```python
from build123d import *

# Parameters (mm, degrees)
SKETCH1_W               = 666.75
SKETCH1_H               = 117.602
BOSS_EXTRUDE1_DEPTH     = 1.5875
CUT_EXTRUDE1_REACH      = 679.044
SKETCH3_W               = 3.175
SKETCH3_H               = 50.8
CUT_EXTRUDE2_DEPTH      = 678.043804388
FILLET1_R               = 2.54
FILLET1_OF_MIRROR1_R    = 2.54
CUT_EXTRUDE3_DEPTH      = 678.043804388
CUT_EXTRUDE3_DEPTH_BACK = 678.043804388
FILLET2_R               = 2.54
CUT_EXTRUDE4_REACH      = 679.044
BOSS_EXTRUDE7_DEPTH     = 1.5875
CUT_EXTRUDE5_REACH      = 679.044
FILLET3_R               = 2.54
BOSS_EXTRUDE9_DEPTH     = 1.5875
CUT_EXTRUDE10_REACH     = 679.044
FILLET4_R               = 2.54
FILLET5_R               = 17.78


with BuildPart() as part:
    # Sketch1 → Boss-Extrude1 (new body)
    with BuildSketch(Plane.XY):
        with Locations((333.375, 58.801)):
            Rectangle(SKETCH1_W, SKETCH1_H)
    extrude(amount=BOSS_EXTRUDE1_DEPTH)

    # Sketch3 → Cut-Extrude1 (cut, up to next)
    with BuildSketch(Plane(origin=(0, 0, 0), x_dir=(-1, 0, 0), z_dir=(0, 0, -1)), mode=Mode.PRIVATE) as cut_extrude1_sk1:
        with Locations((-215.646, 58.801)):
            Rectangle(SKETCH3_W, SKETCH3_H)
    cut_extrude1_tool1 = extrude(cut_extrude1_sk1.sketch, amount=-CUT_EXTRUDE1_REACH, mode=Mode.PRIVATE) & part.part
    # Sketch3 → Cut-Extrude1 (cut, up to next)
    with BuildSketch(Plane(origin=(0, 0, 0), x_dir=(-1, 0, 0), z_dir=(0, 0, -1)), mode=Mode.PRIVATE) as cut_extrude1_sk2:
        with Locations((-451.104, 58.801)):
            Rectangle(SKETCH3_W, SKETCH3_H)
    cut_extrude1_tool2 = extrude(cut_extrude1_sk2.sketch, amount=-CUT_EXTRUDE1_REACH, mode=Mode.PRIVATE) & part.part
    # Sketch3 → Cut-Extrude1 (cut, up to next)
    with BuildSketch(Plane(origin=(0, 0, 0), x_dir=(-1, 0, 0), z_dir=(0, 0, -1)), mode=Mode.PRIVATE) as cut_extrude1_sk3:
        with Locations((-665.1625, 58.801)):
            Rectangle(SKETCH3_W, SKETCH3_H)
    cut_extrude1_tool3 = extrude(cut_extrude1_sk3.sketch, amount=-CUT_EXTRUDE1_REACH, mode=Mode.PRIVATE) & part.part
    # Sketch3 → Cut-Extrude1 (cut, up to next)
    with BuildSketch(Plane(origin=(0, 0, 0), x_dir=(-1, 0, 0), z_dir=(0, 0, -1)), mode=Mode.PRIVATE) as cut_extrude1_sk4:
        with Locations((-1.5875, 58.801)):
            Rectangle(SKETCH3_W, SKETCH3_H)
    cut_extrude1_tool4 = extrude(cut_extrude1_sk4.sketch, amount=-CUT_EXTRUDE1_REACH, mode=Mode.PRIVATE) & part.part
    add(cut_extrude1_tool1.solids().sort_by_distance((215.646, 58.801, 0))[0], mode=Mode.SUBTRACT)
    add(cut_extrude1_tool2.solids().sort_by_distance((451.104, 58.801, 0))[0], mode=Mode.SUBTRACT)
    add(cut_extrude1_tool3.solids().sort_by_distance((665.1625, 58.801, 0))[0], mode=Mode.SUBTRACT)
    add(cut_extrude1_tool4.solids().sort_by_distance((1.5875, 58.801, 0))[0], mode=Mode.SUBTRACT)

    # Sketch4 → Cut-Extrude2 (cut, symmetric)
    with BuildSketch(Plane(origin=(0, 0, 0), x_dir=(-1, 0, 0), z_dir=(0, 0, -1))):
        Polygon((-482.510180694, 104.902), (-633.756319306, 104.902), (-558.13325, 67.310525631), align=None)
        Polygon((-465.3915, 96.392474369), (-465.3915, 21.209525631), (-541.014569306, 58.801), align=None)
        Polygon((-482.510180694, 12.7), (-633.756319306, 12.7), (-558.13325, 50.291474369), align=None)
        Polygon((-650.875, 96.392474369), (-650.875, 21.209525631), (-575.251930694, 58.801), align=None)
    cut_extrude2 = extrude(amount=CUT_EXTRUDE2_DEPTH, both=True, mode=Mode.SUBTRACT)

    # Fillet1
    fillet1_edges = [part.edges().sort_by_distance(p)[0] for p in [
        (650.875, 21.209525631, 0.79375),
        (650.875, 96.392474369, 0.79375),
        (633.756319306, 12.7, 0.79375),
        (558.13325, 50.291474369, 0.79375),
        (482.510180694, 12.7, 0.79375),
        (482.510180694, 104.902, 0.79375),
        (558.13325, 67.310525631, 0.79375),
        (633.756319306, 104.902, 0.79375),
        (541.014569306, 58.801, 0.79375),
        (465.3915, 96.392474369, 0.79375),
        (465.3915, 21.209525631, 0.79375),
        (575.251930694, 58.801, 0.79375),
    ]]
    fillet(fillet1_edges, radius=FILLET1_R)

    # Mirror1: Cut-Extrude2 across plane
    add(cut_extrude2.mirror(Plane(origin=(333.375, 0, 0), x_dir=(0, 0, 1), z_dir=(1, 0, 0))), mode=Mode.SUBTRACT)

    # Fillet1 of Mirror1
    fillet1_of_mirror1_edges = [part.edges().sort_by_distance(p)[0] for p in [
        (15.875, 21.209525631, 0.79375),
        (15.875, 96.392474369, 0.79375),
        (32.993680694, 12.7, 0.79375),
        (108.61675, 50.291474369, 0.79375),
        (184.239819306, 12.7, 0.79375),
        (184.239819306, 104.902, 0.79375),
        (108.61675, 67.310525631, 0.79375),
        (32.993680694, 104.902, 0.79375),
        (125.735430694, 58.801, 0.79375),
        (201.3585, 96.392474369, 0.79375),
        (201.3585, 21.209525631, 0.79375),
        (91.498069306, 58.801, 0.79375),
    ]]
    fillet(fillet1_of_mirror1_edges, radius=FILLET1_OF_MIRROR1_R)

    # Sketch6 → Cut-Extrude3 (cut, two sides: drawn at the far end of the back side and taken through both)
    with BuildSketch(Plane(origin=(0, 0, 0), x_dir=(-1, 0, 0), z_dir=(0, 0, -1)).offset(-CUT_EXTRUDE3_DEPTH_BACK)):
        Polygon((-418.097576662, 12.7), (-248.652423338, 12.7), (-333.375, 50.458496413), align=None)
        Polygon((-436.8165, 21.042503587), (-436.8165, 96.559496413), (-352.093923338, 58.801), align=None)
        Polygon((-418.097576662, 104.902), (-248.652423338, 104.902), (-333.375, 67.143503587), align=None)
        Polygon((-229.9335, 21.042503587), (-229.9335, 96.559496413), (-314.656076662, 58.801), align=None)
    extrude(amount=CUT_EXTRUDE3_DEPTH + CUT_EXTRUDE3_DEPTH_BACK, mode=Mode.SUBTRACT)

    # Fillet2
    fillet2_edges = [part.edges().sort_by_distance(p)[0] for p in [
        (314.656076662, 58.801, 0.79375),
        (229.9335, 96.559496413, 0.79375),
        (229.9335, 21.042503587, 0.79375),
        (418.097576662, 12.7, 0.79375),
        (333.375, 50.458496413, 0.79375),
        (248.652423338, 12.7, 0.79375),
        (352.093923338, 58.801, 0.79375),
        (436.8165, 21.042503587, 0.79375),
        (436.8165, 96.559496413, 0.79375),
        (248.652423338, 104.902, 0.79375),
        (333.375, 67.143503587, 0.79375),
        (418.097576662, 104.902, 0.79375),
    ]]
    fillet(fillet2_edges, radius=FILLET2_R)

    # Sketch7 → Cut-Extrude4 (cut, up to next)
    with BuildSketch(Plane.XY.offset(1.5875), mode=Mode.PRIVATE) as cut_extrude4_sk1:
        Polygon((666.75, 0), (452.6915, 117.602), (666.75, 117.602), align=None)
    cut_extrude4_tool1 = extrude(cut_extrude4_sk1.sketch, amount=-CUT_EXTRUDE4_REACH, mode=Mode.PRIVATE) & part.part
    # Sketch7 → Cut-Extrude4 (cut, up to next)
    with BuildSketch(Plane.XY.offset(1.5875), mode=Mode.PRIVATE) as cut_extrude4_sk2:
        Polygon((0, 117.602), (0, 0), (214.0585, 117.602), align=None)
    cut_extrude4_tool2 = extrude(cut_extrude4_sk2.sketch, amount=-CUT_EXTRUDE4_REACH, mode=Mode.PRIVATE) & part.part
    add(cut_extrude4_tool1.solids().sort_by_distance((595.397167, 78.401333, 1.5875))[0], mode=Mode.SUBTRACT)
    add(cut_extrude4_tool2.solids().sort_by_distance((71.352833, 78.401333, 1.5875))[0], mode=Mode.SUBTRACT)

    # Sketch8 → Boss-Extrude7 (add)
    with BuildSketch(Plane.XY.offset(1.5875)):
        Polygon((452.6915, 117.602), (445.353295325, 104.245041059), (635.099533668, 0), (642.437738342, 13.356958941), align=None)
        Polygon((31.650466332, 0), (24.312261658, 13.356958941), (214.0585, 117.602), (221.396704675, 104.245041059), align=None)
    extrude(amount=-BOSS_EXTRUDE7_DEPTH)

    # Sketch9 → Cut-Extrude5 (cut, up to next)
    with BuildSketch(Plane.XY.offset(1.5875), mode=Mode.PRIVATE) as cut_extrude5_sk1:
        Polygon((465.3915, 92.29335713), (465.3915, 93.236214284), (465.541652204, 93.153721884), align=None)
    cut_extrude5_tool1 = extrude(cut_extrude5_sk1.sketch, amount=-CUT_EXTRUDE5_REACH, mode=Mode.PRIVATE) & part.part
    # Sketch9 → Cut-Extrude5 (cut, up to next)
    with BuildSketch(Plane.XY.offset(1.5875), mode=Mode.PRIVATE) as cut_extrude5_sk2:
        Polygon((201.3585, 93.236214284), (201.208347796, 93.153721884), (201.3585, 92.29335713), align=None)
    cut_extrude5_tool2 = extrude(cut_extrude5_sk2.sketch, amount=-CUT_EXTRUDE5_REACH, mode=Mode.PRIVATE) & part.part
    add(cut_extrude5_tool1.solids().sort_by_distance((465.441551, 92.894431, 1.5875))[0], mode=Mode.SUBTRACT)
    add(cut_extrude5_tool2.solids().sort_by_distance((201.308449, 92.894431, 1.5875))[0], mode=Mode.SUBTRACT)

    # Fillet3
    fillet3_edges = [part.edges().sort_by_distance(p)[0] for p in [
        (534.218957024, 55.422968835, 0.79375),
        (550.482067841, 46.488147941, 0.79375),
        (611.983064985, 12.7, 0.79375),
        (54.766935015, 12.7, 0.79375),
        (116.267932159, 46.488147941, 0.79375),
        (132.531042976, 55.422968835, 0.79375),
        (465.3915, 93.236214284, 0.79375),
        (201.3585, 93.236214284, 0.79375),
    ]]
    fillet(fillet3_edges, radius=FILLET3_R)

    # Sketch13 → Boss-Extrude9 (add)
    with BuildSketch(Plane.XY.offset(1.5875)):
        Polygon((0, 54.934886574), (214.0585, 117.602), (214.0585, 0), (0, 0), align=None)
    extrude(amount=-BOSS_EXTRUDE9_DEPTH)

    # Sketch14 → Cut-Extrude10 (cut, up to next)
    with BuildSketch(Plane.XY.offset(1.5875), mode=Mode.PRIVATE) as cut_extrude10_sk1:
        Polygon((201.3585, 21.092638086), (95.893254571, 69.77525285), (201.3585, 100.650936356), align=None)
    cut_extrude10_tool1 = extrude(cut_extrude10_sk1.sketch, amount=-CUT_EXTRUDE10_REACH, mode=Mode.PRIVATE) & part.part
    # Sketch14 → Cut-Extrude10 (cut, up to next)
    with BuildSketch(Plane.XY.offset(1.5875), mode=Mode.PRIVATE) as cut_extrude10_sk2:
        Polygon((73.642109065, 63.261075374), (183.176821801, 12.7), (12.7, 12.7), (12.7, 45.419849442), align=None)
    cut_extrude10_tool2 = extrude(cut_extrude10_sk2.sketch, amount=-CUT_EXTRUDE10_REACH, mode=Mode.PRIVATE) & part.part
    add(cut_extrude10_tool1.solids().sort_by_distance((166.203418, 63.839609, 1.5875))[0], mode=Mode.SUBTRACT)
    add(cut_extrude10_tool2.solids().sort_by_distance((79.163512, 31.602776, 1.5875))[0], mode=Mode.SUBTRACT)

    # Fillet4
    fillet4_edges = [part.edges().sort_by_distance(p)[0] for p in [
        (201.3585, 100.650936356, 0.79375),
        (201.3585, 21.092638086, 0.79375),
        (95.893254571, 69.77525285, 0.79375),
        (73.642109065, 63.261075374, 0.79375),
        (183.176821801, 12.7, 0.79375),
    ]]
    fillet(fillet4_edges, radius=FILLET4_R)

    # Fillet5
    fillet5_edges = [part.edges().sort_by_distance(p)[0] for p in [
        (12.7, 45.419849442, 0.79375),
        (12.7, 12.7, 0.79375),
    ]]
    fillet(fillet5_edges, radius=FILLET5_R)


solid = part.part
```
The model under review builds one solid part; all positions refer to its coordinate system, in mm. A direction names the side the tool comes from. Round coordinates to 2 decimals unless told otherwise and drop trailing zeros. Write each loop counter-clockwise with the first axis right and the second up, starting at its lowest first coordinate (ties: lowest second). Pieces come first, ordered by that corner, then holes. Notation, with made-up numbers: (-35.75, 35.5) - (4.25, 35.5) arc R14 cw to (4.25, 59.5) - close; hole circle Ø8 at (24, -17.75). An arc over 180 degrees is marked (long way). Answer as CSV lines item,"result". Start each with the question number.
(1) We need section A-A on x = 63.5. State the section outline as (y, z) points.
(2) Draft analysis for pull direction X (two halves, no side actions). For faces 3 (the flat face through (272.011, 39.795, 0.805)), 4 (the flat face through (122.91, 40.52, 0.8)), 5 (the flat face through (561.219, 57.978, 0.805)), 6 (the flat face through (335, 50, 1.588)), state which applies: pulls with the +X half, pulls with the -X half, needs draft (parallel to the pull), parting line crosses it, or undercut.
(3) We need section D-D on z = 0.65. Give the number of separate pieces and of enclosed holes in the cut face, plus the area to 3 significant figures.
(4) For faces 1 (the flat face through (335, 50, 0)), 2 (the flat face through (48.776, 55.981, 0.805)), list the 3-axis set-ups (+Z, -Z, +X, -X, +Y, -Y) from which the entire face can be reached by the end or side of a thin tool; tool diameter is ignored.
(5) We need section B-B on x = 502.5. State the section outline as (y, z) points, plus the area to 3 significant figures.
(6) To check wall thickness, follow line 1 (Y direction, x = 323.5, z = 0.75); line 2 (Y direction, x = 303, z = 0.5); line 3 (Y direction, x = 363, z = 0.3). State the ranges of each line that lie inside material, in increasing order.
(7) For pin 1 Ø0.5 at (x, z) = (452, 0.5) entering from -Y; pin 2 Ø0.5 at (x, z) = (555, 0.5) entering from +Y; pin 3 Ø0.8 at (x, z) = (66.5, 0.5) entering from +Y, all flat-tipped, find the tip position at first contact; note any pin that passes through.
(8) We need section C-C on x = 282. State the section outline as (y, z) points.
Worked answers:
1,outline,"(0, 0) - (12.7, 0) - (12.7, 1.59) - (0, 1.59) - close; (60.29, 0) - (73.52, 0) - (73.52, 1.59) - (60.29, 1.59) - close"
2,face 3,"undercut"
2,face 4,"undercut"
2,face 5,"pulls with the +X half"
2,face 6,"needs draft"
3,separate pieces,"1"
3,enclosed holes,"10"
3,area,"32,100 mm²"
4,face 1,"-Z, +X, -X, +Y, -Y"
4,face 2,"+Z, -Z"
5,outline,"(0, 0) - (12.7, 0) - (12.7, 1.59) - (0, 1.59) - close; (22.64, 0) - (39.66, 0) - (39.66, 1.59) - (22.64, 1.59) - close; (72.85, 0) - (90.24, 0) - (90.24, 1.59) - (72.85, 1.59) - close"
5,area,"74.8 mm²"
6,line 1,"0 to 12.7, 46.06 to 71.54, 104.9 to 117.6"
6,line 2,"0 to 12.7, 36.92 to 53.61, 64 to 80.68, 104.9 to 117.6"
6,line 3,"0 to 12.7, 37.26 to 53.94, 63.66 to 80.35, 104.9 to 117.6"
7,pin 1,"y = 0"
7,pin 2,"y = 61.53"
7,pin 3,"y = 74.52"
8,outline,"(0, 0) - (12.7, 0) - (12.7, 1.59) - (0, 1.59) - close; (27.56, 0) - (44.25, 0) - (44.25, 1.59) - (27.56, 1.59) - close; (73.35, 0) - (90.04, 0) - (90.04, 1.59) - (73.35, 1.59) - close; (104.9, 0) - (117.6, 0) - (117.6, 1.59) - (104.9, 1.59) - close"
